Read the model definition and answer for the solid it produces. Units are mm, in the model's axes. Face numbers are marked on the shaded views. A direction names the side the tool comes from. Coordinates: 2 decimals unless noted, no trailing zeros. Write each loop counter-clockwise with the first axis right and the second up, starting at its lowest first coordinate (ties: lowest second). Pieces come first, ordered by that corner, then holes.
(1) Given pin 1 (12 mm diameter, centred on y = -61.5, z = 115.5, fed in from +X); pin 2 (4 mm diameter, centred on x = 14, y = 68.5, fed in from -Z), each flat-ended and moving along its own axis, determine where each tip first touches the part or whether it passes through.
(2) Section B-B on y = 124.5 is taken. Write down the section's boundary in (x, z).
(3) Find the intervals of material crossed by probe 1 along X at (y, z) = (-44, 123); probe 2 along Z at (x, y) = (51, -117.5), in increasing order.
(4) Section C-C on x = 22 is taken. Write down the section's boundary in (y, z).
(5) Which of the six approach directions +Z, -Z, +X, -X, +Y, -Y give full straight-line access (tool end or side, diameter ignored) to the marked faces 1 and 2?
(6) Section A-A on z = 0 is taken. Write down the section's boundary in (x, y).
from build123d import *

# Parameters (mm, degrees)
F0_W     = 400.146693
F0_H     = 364.072472
F2_DEPTH = 76.2
F1_R     = 29.21
F3_DEPTH = 76.2


with BuildPart() as f2:
    # F0 (on Right) → F2 (new body)
    with BuildSketch(Plane.YZ):
        with Locations((-8.979843, 58.667138)):
            Rectangle(F0_W, F0_H)
    extrude(amount=-F2_DEPTH)

    # F1 (on face) → F3 (join)
    with BuildSketch(Plane.YZ):
        with Locations((-134.976578, 0)):
            Circle(F1_R)
        with Locations((101.243422, 89.998201)):
            Circle(F1_R)
    extrude(amount=F3_DEPTH)


solid = f2.part
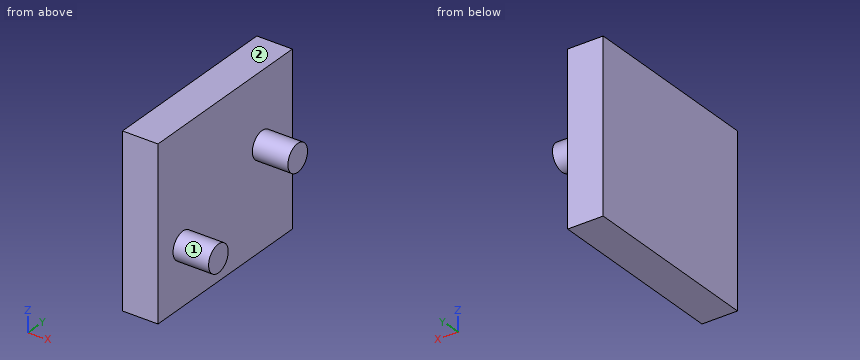
Response:
1. pin 1: stops at x = 0
1. pin 2: passes through
2. outline: (-76.2, -123.37) - (0, -123.37) - (0, 72.32) - (76.2, 72.32) - (76.2, 107.67) - (0, 107.67) - (0, 240.7) - (-76.2, 240.7) - close
3. probe 1: x = -76.2 to 0
3. probe 2: z = -23.4 to 23.4
4. outline: circle Ø58.42 at (-134.98, 0); circle Ø58.42 at (101.24, 90)
5. face 1: +X
5. face 2: +Z, +X, -X, +Y, -Y
6. outline: (-76.2, -209.05) - (0, -209.05) - (0, -164.19) - (76.2, -164.19) - (76.2, -105.77) - (0, -105.77) - (0, 191.09) - (-76.2, 191.09) - close
